Read the model definition and answer for the solid it produces. Units are mm, in the model's axes. A direction names the side the tool comes from. Coordinates: 2 decimals unless noted, no trailing zeros. Write each loop counter-clockwise with the first axis right and the second up, starting at its lowest first coordinate (ties: lowest second). Pieces come first, ordered by that corner, then holes. Notation, with made-up numbers: (80.5, 21.25) -> (122.5, 21.25) arc R27 ccw to (122.5, 48.25) -> close; hole circle Ø9 at (16.5, 54.25). An arc over 180 degrees is marked (long way). Use CSV: the item, a comma, the result in double quotes.
from build123d import *

# Parameters (mm, degrees)
F0_R     = 31.75
F2_DEPTH = 152.4
F1_R     = 19.05
F3_DEPTH = 152.4
F4_R     = 9.525
F5_DEPTH = 38.1
F6_W     = 38.1
F6_H     = 12.7
F7_DEPTH = 50.8


with BuildPart() as f2:
    # F0 (on Right) → F2 (new body)
    with BuildSketch(Plane.YZ):
        with Locations((0.1902006916, -0.0633993695)):
            Circle(F0_R)
    extrude(amount=F2_DEPTH)

    # F1 (on Right) → F3 (cut)
    with BuildSketch(Plane.YZ):
        with Locations((0.1902006916, 0.4437955504)):
            Circle(F1_R)
    extrude(amount=F3_DEPTH, mode=Mode.SUBTRACT)

    # F4 (on Front) → F5 (cut, symmetric)
    with BuildSketch(Plane.XZ):
        with Locations((19.0424583852, 0.2906440059)):
            Circle(F4_R)
    extrude(amount=F5_DEPTH, both=True, mode=Mode.SUBTRACT)

    # F6 (on Top) → F7 (cut)
    with BuildSketch(Plane.XY):
        with Locations((17.8630856547, 3.4606340123)):
            Rectangle(F6_W, F6_H)
    extrude(amount=F7_DEPTH, mode=Mode.SUBTRACT)


solid = f2.part
1. A tool of negligible diameter and unlimited length cuts with its end or side. For faces 4 (the cylindrical face through (28.13, -24, 3.15)), 5 (the flat face through (18, -2.889, 25)), from which of +Z, -Z, +X, -X, +Y, -Y can it reach the whole face along a straight path? Write none if from no direction.
Solutions:
face 4,"+Y, -Y"
face 5,"+Z, -X"
2. A cutting plane is placed at B-B (y = -14). Give the vertices of the cut face in (x, z).
Solutions:
outline,"(0, -28.47) -> (152.4, -28.47) -> (152.4, -12.27) -> (0, -12.27) -> close; (0, 13.15) -> (152.4, 13.15) -> (152.4, 28.34) -> (0, 28.34) -> close"
3. A cutting plane is placed at C-C (x = 14). Give the vertices of the cut face in (y, z), and give its area (3 significant figures).
Solutions:
outline,"(-30.61, -7.79) arc R31.75 ccw to (30.99, -7.79) -> (17.37, -7.79) arc R19.05 cw to (-16.99, -7.79) -> close; (-30.42, 8.37) -> (-17.13, 8.37) arc R19.05 cw to (-2.89, 19.24) -> (-2.89, 31.54) arc R31.75 ccw to start; (9.81, 16.89) arc R19.05 cw to (17.51, 8.37) -> (30.8, 8.37) arc R31.75 ccw to (9.81, 30.19) -> close"
area,"1,450 mm^2"
4. Each of these flat-tipped pins is pushed along its axis until it touches: pin 1 Ø4 at (x, z) = (89.5, -20) entering from +Y; pin 2 Ø5 at (x, y) = (124, 1) entering from -Z; pin 3 Ø13.5 at (x, z) = (22.5, 26) entering from +Y; pin 4 Ø17 at (x, z) = (19.04, 0.29) entering from -Y. Where does it stop, or does it pass through?
Solutions:
pin 1,"stops at y = 26.39"
pin 2,"stops at z = -31.81"
pin 3,"stops at y = 25.39"
pin 4,"passes through"
5. A cutting plane is placed at A-A (z = -11.5). Give the vertices of the cut face in (x, y).
Solutions:
outline,"(0, -29.43) -> (152.4, -29.43) -> (152.4, -14.65) -> (0, -14.65) -> close; (0, 15.03) -> (152.4, 15.03) -> (152.4, 29.81) -> (0, 29.81) -> close"
6. Find the intervals of material crossed by line 1 along Z through (x, y) = (135, 0); line 2 along Y through (x, z) = (40, 1); line 3 along X through (y, z) = (20, -5.5), in increasing order.
Solutions:
line 1,"z = -31.81 to -18.61, 19.49 to 31.69"
line 2,"y = -31.54 to -18.85, 19.23 to 31.92"
line 3,"x = 0 to 11.48, 26.61 to 152.4"
7. A cutting plane is placed at D-D (z = 3). Give the vertices of the cut face in (x, y), and give its area (3 significant figures).
Solutions:
outline,"(0, -31.41) -> (9.91, -31.41) -> (9.91, -18.69) -> (0, -18.69) -> close; (0, 19.07) -> (9.91, 19.07) -> (9.91, 31.79) -> (0, 31.79) -> close; (28.17, -31.41) -> (152.4, -31.41) -> (152.4, -18.69) -> (28.17, -18.69) -> close; (28.17, 19.07) -> (152.4, 19.07) -> (152.4, 31.79) -> (28.17, 31.79) -> close"
area,"3,410 mm^2"
8. For a pull along Y with two mould halves and no side action, classify faces 1 (the cylindrical face through (75.13, 29.52, -12.22)), 2 (the cylindrical face through (23.44, 24.16, -8.16)), 3 (the cylindrical face through (75.133, -3.939, -18.153)) as pulls with the +Y half, pulls with the -Y half, needs draft (parallel to the pull), parting line crosses it, or undercut.
Solutions:
face 1,"parting line crosses it"
face 2,"needs draft"
face 3,"undercut"
